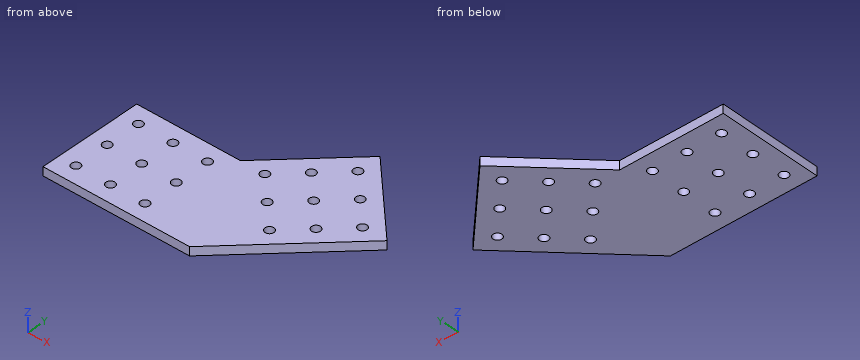
Autodesk Inventor part; units mm, degrees
ref_plane "YZ Plane" through (0, 0, 0) normal (1, 0, 0) x (0, 1, 0)
ref_plane "XZ Plane" through (0, 0, 0) normal (0, 1, 0) x (-1, 0, 0)
ref_plane "XY Plane" through (0, 0, 0) normal (0, 0, 1) x (1, 0, 0)
sketch "Sketch1" plane through (0, 0, 0) normal (0, 0, 1) x (1, 0, 0)
  line L0 (76.2, 76.2) -> (0, 76.2)
  line L1 (0, 76.2) -> (0, 0)
  line L2 (76.2, 76.2) -> (130.0815, 130.0815)
  line L3 (130.0815, 130.0815) -> (183.9631, 76.2)
  line L4 (0, 0) -> (107.7631, 0)
  line L5 (183.9631, 76.2) -> (107.7631, 0)
  circle A0 centre (12.7, 12.7) radius 3.2512
  circle A1 centre (12.7, 38.1) radius 3.2512
  circle A2 centre (12.7, 63.5) radius 3.2512
  circle A3 centre (38.1, 12.7) radius 3.2512
  circle A4 centre (38.1, 38.1) radius 3.2512
  circle A5 centre (38.1, 63.5) radius 3.2512
  circle A6 centre (63.5, 12.7) radius 3.2512
  circle A7 centre (63.5, 38.1) radius 3.2512
  circle A8 centre (63.5, 63.5) radius 3.2512
  circle A9 centre (166.0026, 76.2) radius 3.2512
  circle A10 centre (148.042, 94.1605) radius 3.2512
  circle A11 centre (130.0815, 112.121) radius 3.2512
  circle A12 centre (148.042, 58.2395) radius 3.2512
  circle A13 centre (130.0815, 76.2) radius 3.2512
  circle A14 centre (112.121, 94.1605) radius 3.2512
  circle A15 centre (130.0815, 40.279) radius 3.2512
  circle A16 centre (112.121, 58.2395) radius 3.2512
  circle A17 centre (94.1605, 76.2) radius 3.2512
  dimension "d5" = 76.2
  dimension "d7" = 76.2
  dimension "d8" = 135
  dimension "d11" = 76.2
  dimension "d12" = 76.2
  dimension "d13" = 76.2
  dimension "d14" = 6.5024
  dimension "d15" = 12.7
  dimension "d16" = 12.7
  dimension "d19" = 25.4
  dimension "d22" = 25.4
  dimension "d25" = 6.5024
  dimension "d26" = 12.7
  dimension "d27" = 12.7
  dimension "d30" = 25.4
  dimension "d33" = 25.4
extrude "Extrusion1" add sketch "Sketch1" along normal blind 6.35
properties part number "3x3 V plate"
The listing builds one solid part. Answer for the finished solid, in the listing's coordinates (mm). Round coordinates to 2 decimals unless told otherwise and drop trailing zeros. Write each loop counter-clockwise with the first axis right and the second up, starting at its lowest first coordinate (ties: lowest second). Pieces come first, ordered by that corner, then holes. Notation, with made-up numbers: (5, -24) -> (39, -24) arc R22 cw to (39, 1) -> close; hole circle Ø8 at (22.25, 84.25). An arc over 180 degrees is marked (long way). Use CSV: the item, a comma, the result in double quotes. Start each with the question number.
(1) Section D-D on x = 94 is taken. Give the vertices of the cut face in (y, z).
(2) This flat-tipped pin is pushed along its axis until it touches: pin 1 (3 mm diameter, centred on x = 55.5, z = 3, fed in from +Y). Where does it stop, or does it pass through?
(3) Consider L1, parallel to Y at x = 38.1, z = 3; L2, parallel to X at y = 14, z = 0.75; L3, parallel to X at y = 13.5, z = 4. Determine where each line is inside the solid, lowest interval first. Write a range as from..to.
(4) Section C-C on z = 5 is taken. Count the separate pieces of the cut face and the enclosed holes in it, then the cut area to 3 significant figures.
(5) Section A-A on x = 12.7 is taken. Give the vertices of the cut face in (y, z), then the cut area to 3 significant figures.
(6) Section B-B on y = 63.5 is taken. Give the vertices of the cut face in (x, z).
A:
1,outline,"(0, 0) -> (72.95, 0) -> (72.95, 6.35) -> (0, 6.35) -> close; (79.45, 0) -> (94, 0) -> (94, 6.35) -> (79.45, 6.35) -> close"
2,pin 1,"stops at y = 76.2"
3,L1,"y = 0..9.45, 15.95..34.85, 41.35..60.25, 66.75..76.2"
3,L2,"x = 0..9.72, 15.68..35.12, 41.08..60.52, 66.48..121.76"
3,L3,"x = 0..9.55, 15.85..34.95, 41.25..60.35, 66.65..121.26"
4,separate pieces,"1"
4,enclosed holes,"18"
4,area,"13,400 mm²"
5,outline,"(0, 0) -> (9.45, 0) -> (9.45, 6.35) -> (0, 6.35) -> close; (15.95, 0) -> (34.85, 0) -> (34.85, 6.35) -> (15.95, 6.35) -> close; (41.35, 0) -> (60.25, 0) -> (60.25, 6.35) -> (41.35, 6.35) -> close; (66.75, 0) -> (76.2, 0) -> (76.2, 6.35) -> (66.75, 6.35) -> close"
5,area,"360 mm²"
6,outline,"(0, 0) -> (9.45, 0) -> (9.45, 6.35) -> (0, 6.35) -> close; (15.95, 0) -> (34.85, 0) -> (34.85, 6.35) -> (15.95, 6.35) -> close; (41.35, 0) -> (60.25, 0) -> (60.25, 6.35) -> (41.35, 6.35) -> close; (66.75, 0) -> (171.26, 0) -> (171.26, 6.35) -> (66.75, 6.35) -> close"
